Design review of the part built by this model. Coordinates are the model's own, in mm. Face numbers are marked on the shaded views. A direction names the side the tool comes from. Coordinates: 2 decimals unless noted, no trailing zeros. Loops run counter-clockwise (first coordinate to the right, second up) from the corner with the lowest first, then second, coordinate; pieces in that order, holes last. Notation, with made-up numbers: (-33.5, -33.5) - (25.5, -33.5) arc R23 ccw to (25.5, 5.5) - close; hole circle Ø9 at (32, 65.5). An arc over 180 degrees is marked (long way). Return JSON: item names as keys, results as strings. Group by question number.
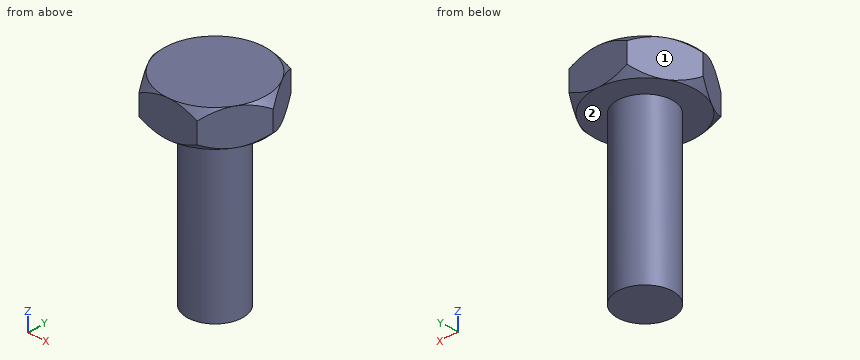
from build123d import *

# Parameters (mm, degrees)
BOSS_EXTRUDE1_DEPTH = 3.895
SKETCH2_OUTSIDE_W   = 51.796
SKETCH2_OUTSIDE_H   = 48.402
SKETCH2_OUTSIDE_R   = 10.969655115
CUT_EXTRUDE1_DEPTH  = 8.79
CUT_EXTRUDE1_TAPER  = 45
SKETCH3_R           = 6
BOSS_EXTRUDE2_DEPTH = 35.5


with BuildPart() as part:
    # Sketch1 → Boss-Extrude1 (new body, symmetric)
    with BuildSketch(Plane.XY):
        Polygon((-6.333333333, 10.969655115), (-12.666666667, 0), (-6.333333333, -10.969655115), (6.333333333, -10.969655115), (12.666666667, 0), (6.333333333, 10.969655115), align=None)
    extrude(amount=BOSS_EXTRUDE1_DEPTH, both=True)

    # Sketch2 outside → Cut-Extrude1 (cut, through all)
    with BuildSketch(Plane.XY.offset(3.895)):
        Rectangle(SKETCH2_OUTSIDE_W, SKETCH2_OUTSIDE_H)
        Circle(SKETCH2_OUTSIDE_R, mode=Mode.SUBTRACT)
    cut_extrude1 = extrude(amount=-CUT_EXTRUDE1_DEPTH, taper=CUT_EXTRUDE1_TAPER, mode=Mode.SUBTRACT)

    # Mirror1: Cut-Extrude1 across plane
    add(cut_extrude1.mirror(Plane.XY), mode=Mode.SUBTRACT)

    # Sketch3 → Boss-Extrude2 (add)
    with BuildSketch(Plane(origin=(0, 0, -3.895), x_dir=(-1, 0, 0), z_dir=(0, 0, -1))):
        Circle(SKETCH3_R)
    extrude(amount=BOSS_EXTRUDE2_DEPTH)


solid = part.part
Item 1: For P1, Ø12, axis at y = -3, z = -30, coming from the -X side; P2, Ø3, axis at y = -1.5, z = -26.5, coming from the +X side; P3, Ø4, axis at x = -4, z = -12.5, coming from the -Y side; P4, Ø2, axis at x = -8.5, z = -16, coming from the +Y side, all flat-tipped, find the tip position at first contact; note any pin that passes through.
Item 2: To check wall thickness, follow line 1 (Z direction, x = -9.75, y = 3) (3 decimals); line 2 (Y direction, x = -5.25, z = -22); line 3 (Y direction, x = 5, z = -26.5). State the ranges of each line that lie inside material, in increasing order. Write a range as from..to.
Item 3: For the marked faces 1 and 2, list the 3-axis set-ups (+Z, -Z, +X, -X, +Y, -Y) from which the entire face can be reached by the end or side of a thin tool; tool diameter is ignored.
Item 4: Add section A-A (z = -1). State the section outline as (x, y) points, then the cut area to 3 significant figures.
Item 5: Add section B-B (z = -23). State the section outline as (x, y) points, then the cut area to 3 significant figures.
Answers below:
{
 "1": {"P1": "stops at x = -6", "P2": "stops at x = 6", "P3": "stops at y = -5.66", "P4": "passes through"},
 "2": {"line 1": "z = -3.895..3.895", "line 2": "y = -2.9..2.9", "line 3": "y = -3.32..3.32"},
 "3": {"face 1": "+Z, -Z, -X, +Y", "face 2": "-Z"},
 "4": {"outline": "(-12.67, 0) - (-6.33, -10.97) - (6.33, -10.97) - (12.67, 0) - (6.33, 10.97) - (-6.33, 10.97) - close", "area": "417 mm^2"},
 "5": {"outline": "circle Ø12 at (0, 0)", "area": "113 mm^2"}
}
